```python
from build123d import *

# Parameters (mm, degrees)
SKETCH1_W                       = 22.5
SKETCH1_H                       = 20
BOSS_EXTRUDE1_DEPTH             = 5
CBORE_FOR_M2_SHCS1_D            = 2.2
CBORE_FOR_M2_SHCS1_CBORE_D      = 4.4
CBORE_FOR_M2_SHCS1_CBORE_DEPTH  = 2
TAP_DRILL_FOR_M2X0_4_TAP1_D     = 3.3
TAP_DRILL_FOR_M2X0_4_TAP1_DEPTH = 6.008579979
TAP_DRILL_FOR_M2X0_4_TAP1_TIP   = 0.991420021
SKETCH9_W                       = 5
SKETCH9_H                       = 20
BOSS_EXTRUDE2_DEPTH             = 5
F_3_0MM_DOWEL_HOLE1_D           = 3
CUT_EXTRUDE1_DEPTH              = 2.4


with BuildPart() as part:
    # Sketch1 → Boss-Extrude1 (new body)
    with BuildSketch(Plane.XY):
        Rectangle(SKETCH1_W, SKETCH1_H)
    extrude(amount=BOSS_EXTRUDE1_DEPTH)

    # CBORE for M2 SHCS1 (through all)
    with Locations(Plane.XY.offset(5)):
        with Locations((4, 6), (-4, -6), (-4, 6), (4, -6)):
            CounterBoreHole(CBORE_FOR_M2_SHCS1_D / 2, CBORE_FOR_M2_SHCS1_CBORE_D / 2, CBORE_FOR_M2_SHCS1_CBORE_DEPTH)

    # Tap Drill for M2x0.4 Tap1
    with Locations(Plane(origin=(0, 10, 0), x_dir=(1, 0, 0), z_dir=(0, 1, 0))):
        with Locations((8, -1.59), (-8, -1.59)):
            Hole(TAP_DRILL_FOR_M2X0_4_TAP1_D / 2, depth=TAP_DRILL_FOR_M2X0_4_TAP1_DEPTH)
            with Locations((0, 0, -(TAP_DRILL_FOR_M2X0_4_TAP1_DEPTH + TAP_DRILL_FOR_M2X0_4_TAP1_TIP / 2))):  # 118° drill point
                Cone(0, TAP_DRILL_FOR_M2X0_4_TAP1_D / 2, TAP_DRILL_FOR_M2X0_4_TAP1_TIP, mode=Mode.SUBTRACT)

    # Sketch9 → Boss-Extrude2 (add)
    with BuildSketch(Plane.XY.offset(5)):
        with Locations((-13.75, 0)):
            Rectangle(SKETCH9_W, SKETCH9_H)
        with Locations((13.75, 0)):
            Rectangle(SKETCH9_W, SKETCH9_H)
    extrude(amount=-BOSS_EXTRUDE2_DEPTH)

    # Ø3.0mm Dowel Hole1 (through all)
    with Locations(Plane.XY.offset(5)):
        with Locations((0, 0), (-13, 6), (-13, -6), (13, -6), (13, 6)):
            Hole(F_3_0MM_DOWEL_HOLE1_D / 2)

    # Sketch12 → Cut-Extrude1 (cut)
    with BuildSketch(Plane(origin=(0, 0, 0), x_dir=(-1, 0, 0), z_dir=(0, 0, -1))):
        Polygon((-13, 2.824573519), (-10.25, 4.41228676), (-10.25, 7.58771324), (-13, 9.175426481), (-15.75, 7.58771324), (-15.75, 4.41228676), align=None)
        Polygon((0, -3.175426481), (2.75, -1.58771324), (2.75, 1.58771324), (0, 3.175426481), (-2.75, 1.58771324), (-2.75, -1.58771324), align=None)
        Polygon((13, 2.824573519), (15.75, 4.41228676), (15.75, 7.58771324), (13, 9.175426481), (10.25, 7.58771324), (10.25, 4.41228676), align=None)
        Polygon((13, -2.824573519), (10.25, -4.41228676), (10.25, -7.58771324), (13, -9.175426481), (15.75, -7.58771324), (15.75, -4.41228676), align=None)
        Polygon((-13, -2.824573519), (-15.75, -4.41228676), (-15.75, -7.58771324), (-13, -9.175426481), (-10.25, -7.58771324), (-10.25, -4.41228676), align=None)
    extrude(amount=-CUT_EXTRUDE1_DEPTH, mode=Mode.SUBTRACT)


solid = part.part
```
Geometry check sheet. Reference: the model listing, model coordinates, mm. A direction names the side the tool comes from. Give positions to 0.01 mm unless a question says otherwise; leave off trailing zeros. Write each loop counter-clockwise with the first axis right and the second up, starting at its lowest first coordinate (ties: lowest second). Pieces come first, ordered by that corner, then holes.
1) Access from +Z, -Z, +X, -X, +Y, -Y to the whole of each face (thin tool, end or side, straight path). Record for faces 1 (the flat face through (-16.25, 0, 3)), 2 (the flat face through (-10.25, 6, 1)), 3 (the flat face through (-5, 7, 3)).
2) Release check for a two-part mould opening along Z. For faces 4 (the cylindrical face through (-5.016, 5.579, 1.479)), 5 (the cylindrical face through (8.07, 6.95, 3.24)), 6 (the flat face through (-11.7, -7.4, 2.4)) record: pulls with the +Z half, pulls with the -Z half, needs draft (parallel to the pull), parting line crosses it, or undercut.
3) Section check C-C, the plane x = -13.5. Record the boundary of the cut face in (y, z), and give its area (3 significant figures).
4) Section check D-D, the plane y = 6. State how many separate pieces and enclosed holes the cut face has, and give its area (3 significant figures).
5) Material ranges on L1, parallel to Y at x = -4, z = 3.7; L2, parallel to X at y = 5, z = 4.8; L3, parallel to X at y = -8.5, z = 1.95, recorded low to high.
6) Gauge pin test, flat ends, axial feed: pin 1 (2 mm diameter, centred on x = -4, y = 1, fed in from -Z); pin 2 (3.5 mm diameter, centred on x = 4, y = 6, fed in from +Z); pin 3 (2 mm diameter, centred on x = 0, y = 1, fed in from -Z). Record the tip position at first contact, or that the pin passes through.
7) Section check A-A, the plane y = 0. Record the boundary of the cut face in (x, z).
8) Section check B-B, the plane x = -4. Record the boundary of the cut face in (y, z).
Computed:
1. face 1: +Z, -Z, -X, +Y, -Y
1. face 2: -Z
1. face 3: +Z
2. face 4: needs draft
2. face 5: undercut
2. face 6: pulls with the -Z half
3. outline: (-10, 0) - (-8.89, 0) - (-8.89, 2.4) - (-7.41, 2.4) - (-7.41, 5) - (-10, 5) - close; (-4.59, 2.4) - (-3.11, 2.4) - (-3.11, 0) - (3.11, 0) - (3.11, 2.4) - (4.59, 2.4) - (4.59, 5) - (-4.59, 5) - close; (7.41, 2.4) - (8.89, 2.4) - (8.89, 0) - (10, 0) - (10, 5) - (7.41, 5) - close
3. area: 57.6 mm2
4. separate pieces: 5
4. enclosed holes: 0
4. area: 72.7 mm2
5. L1: y = -10 to -8.2, -3.8 to 3.8, 8.2 to 10
5. L2: x = -16.25 to -14.12, -11.88 to -5.96, -2.04 to 2.04, 5.96 to 11.88, 14.12 to 16.25
5. L3: x = -16.25 to -14.17, -11.83 to 11.83, 14.17 to 16.25
6. pin 1: stops at z = 0
6. pin 2: stops at z = 3
6. pin 3: stops at z = 2.4
7. outline: (-16.25, 0) - (-2.75, 0) - (-2.75, 2.4) - (-1.5, 2.4) - (-1.5, 5) - (-16.25, 5) - close; (1.5, 2.4) - (2.75, 2.4) - (2.75, 0) - (16.25, 0) - (16.25, 5) - (1.5, 5) - close
8. outline: (-10, 0) - (-7.1, 0) - (-7.1, 3) - (-8.2, 3) - (-8.2, 5) - (-10, 5) - close; (-4.9, 0) - (4.9, 0) - (4.9, 3) - (3.8, 3) - (3.8, 5) - (-3.8, 5) - (-3.8, 3) - (-4.9, 3) - close; (7.1, 0) - (10, 0) - (10, 5) - (8.2, 5) - (8.2, 3) - (7.1, 3) - close
